For this review, use the dimensioned drawing (mm, ordinates from the lowest corner) and the shaded views. A direction names the side the tool comes from. Round coordinates to 2 decimals unless told otherwise and drop trailing zeros. Order: outer loops, then holes, each group sorted by start corner. A loop starts at its lowest first (then second) coordinate and runs counter-clockwise, first axis right, second up. Notation, with made-up numbers: (71, 81.25) -> (102, 81.25) arc R22 cw to (102, 104.25) -> close; hole circle Ø5 at (15.25, 13.25). An arc over 180 degrees is marked (long way). Answer in a Markdown table with one row per item.
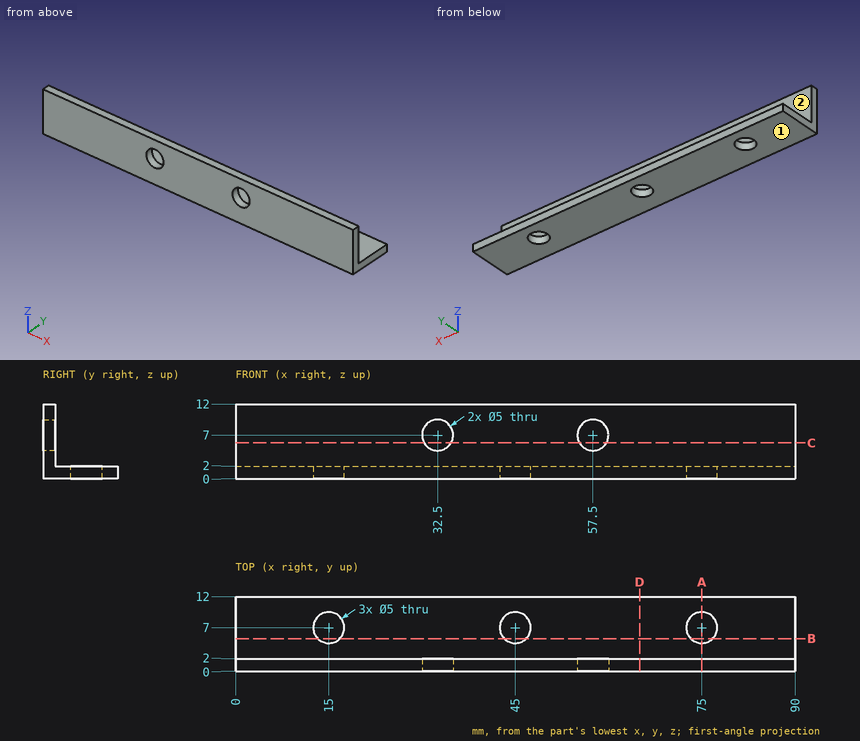
Q1. Take a section at D-D, the plane x = 65. Write out the cut boundary in (y, z).
Answer key:
| item | result |
|---|---|
| outline | (0, 0) -> (12, 0) -> (12, 2) -> (2, 2) -> (2, 12) -> (0, 12) -> close |
Q2. Take a section at B-B, the plane y = 5.25. Write out the cut boundary in (x, z), then the cut area to 3 significant figures.
Answer key:
| item | result |
|---|---|
| outline | (0, 0) -> (13.21, 0) -> (13.21, 2) -> (0, 2) -> close; (16.79, 0) -> (43.21, 0) -> (43.21, 2) -> (16.79, 2) -> close; (46.79, 0) -> (73.21, 0) -> (73.21, 2) -> (46.79, 2) -> close; (76.79, 0) -> (90, 0) -> (90, 2) -> (76.79, 2) -> close |
| area | 159 mm^2 |
Q3. Take a section at C-C, the plane z = 5.75. Write out the cut boundary in (x, y).
Answer key:
| item | result |
|---|---|
| outline | (0, 0) -> (30.33, 0) -> (30.33, 2) -> (0, 2) -> close; (34.67, 0) -> (55.33, 0) -> (55.33, 2) -> (34.67, 2) -> close; (59.67, 0) -> (90, 0) -> (90, 2) -> (59.67, 2) -> close |
Q4. To check wall thickness, follow probe 1 along X at (y, z) = (7, 1.4); probe 2 along X at (y, z) = (0.9, 7); probe 3 along X at (y, z) = (9.25, 1.75). State the ranges of each line that lie inside material, in increasing order.
Answer key:
| item | result |
|---|---|
| probe 1 | x = 0 to 12.5, 17.5 to 42.5, 47.5 to 72.5, 77.5 to 90 |
| probe 2 | x = 0 to 30, 35 to 55, 60 to 90 |
| probe 3 | x = 0 to 13.91, 16.09 to 43.91, 46.09 to 73.91, 76.09 to 90 |
Q5. Tool access review of the marked faces 1 and 2: name each direction out of +Z, -Z, +X, -X, +Y, -Y from which nothing blocks a thin tool from reaching the whole face with its end or side.
Answer key:
| item | result |
|---|---|
| face 1 | -Z, +X, -X, +Y, -Y |
| face 2 | +Z, +X, -X, +Y |
Q6. Take a section at A-A, the plane x = 75. Write out the cut boundary in (y, z).
Answer key:
| item | result |
|---|---|
| outline | (0, 0) -> (4.5, 0) -> (4.5, 2) -> (2, 2) -> (2, 12) -> (0, 12) -> close; (9.5, 0) -> (12, 0) -> (12, 2) -> (9.5, 2) -> close |
Q7. Clearance check with flat-ended pins moving along their axes: pin 1 Ø3 at (y, z) = (10.5, 5) entering from -X; pin 2 Ø3 at (x, y) = (66, 7.5) entering from +Z; pin 3 Ø3 at (x, z) = (29.5, 4) entering from +Y. State where each tip first meets the part, or that it passes through.
Answer key:
| item | result |
|---|---|
| pin 1 | passes through |
| pin 2 | stops at z = 2 |
| pin 3 | stops at y = 2 |
